from build123d import *

# Parameters (mm, degrees)
CROQUIS1_R              = 10.5
SALIENTE_EXTRUIR1_DEPTH = 10


with BuildPart() as part:
    # Croquis1 → Saliente-Extruir1 (new body)
    with BuildSketch(Plane(origin=(0, 0, 0), x_dir=(0, 0, -1), z_dir=(1, 0, 0))):
        with BuildLine():
            Line((-18.5, 12.5), (18.5, 12.5))
            ThreePointArc((18.5, 12.5), (30.713875068, 2.659183298), (23.696629213, -11.36859907))
            ThreePointArc((23.696629213, -11.36859907), (0, -16.52778731), (-23.696629213, -11.36859907))
            ThreePointArc((-23.696629213, -11.36859907), (-30.713875068, 2.659183298), (-18.5, 12.5))
        make_face()
        with Locations((18.5, 0)):
            Circle(CROQUIS1_R, mode=Mode.SUBTRACT)
        with Locations((-18.5, 0)):
            Circle(CROQUIS1_R, mode=Mode.SUBTRACT)
        with BuildLine():
            Line((-6, -6.020797289), (-6, 6.020797289))
            ThreePointArc((-6, 6.020797289), (0, 8.5), (6, 6.020797289))
            Line((6, 6.020797289), (6, -6.020797289))
            ThreePointArc((6, -6.020797289), (0, -8.5), (-6, -6.020797289))
        make_face(mode=Mode.SUBTRACT)
    extrude(amount=SALIENTE_EXTRUIR1_DEPTH)


solid = part.part
Check sheet for the modelled part. Datum: model origin and axes. Units: mm. A direction names the side the tool comes from. Round coordinates to 2 decimals unless told otherwise and drop trailing zeros. Order: outer loops, then holes, each group sorted by start corner. A loop starts at its lowest first (then second) coordinate and runs counter-clockwise, first axis right, second up.
Q1. Cross-section at B-B, the plane x = 8.75. Enter the section's corners in (y, z).
Filled sheet:
outline: (-11.37, -23.7) arc R12.5 ccw to (12.5, -18.5) - (12.5, 18.5) arc R12.5 ccw to (-11.37, 23.7) arc R57 ccw to start; hole circle Ø21 at (0, -18.5); hole circle Ø21 at (0, 18.5); hole (-6.02, -6) - (6.02, -6) arc R8.5 ccw to (6.02, 6) - (-6.02, 6) arc R8.5 ccw to start
Q2. Draft check along Z on faces 1 (the face through (4.9, 8.5, 0.1)), 2 (the face through (4.93, 2.43, 30.76)), 3 (the face through (10, -2, -7)). Enter one of: pulls with the +Z half, pulls with the -Z half, needs draft (parallel to the pull), parting line crosses it, or undercut.
Filled sheet:
face 1: undercut
face 2: pulls with the +Z half
face 3: needs draft
Q3. Cross-section at A-A, the plane y = 0. Enter the section's corners in (x, z), plus the area to 3 significant figures.
Filled sheet:
outline: (0, -31) - (10, -31) - (10, -29) - (0, -29) - close; (0, -8) - (10, -8) - (10, -6) - (0, -6) - close; (0, 6) - (10, 6) - (10, 8) - (0, 8) - close; (0, 29) - (10, 29) - (10, 31) - (0, 31) - close
area: 80.0 mm2
Q4. Scan lines: L1, parallel to Z at x = 3.5, y = 4.75; L2, parallel to Z at x = 7.5, y = -9.25; L3, parallel to Y at x = 8.75, z = 0. Record each from-to range of solid material in increasing order.
Filled sheet:
L1: z = -30.06 to -27.86, -9.14 to -6, 6 to 9.14, 27.86 to 30.06
L2: z = -26.91 to -23.47, -13.53 to 13.53, 23.47 to 26.91
L3: y = -16.53 to -8.5, 8.5 to 12.5
Q5. Cross-section at C-C, the plane z = -5. Enter the section's corners in (x, y).
Filled sheet:
outline: (0, -16.31) - (10, -16.31) - (10, -6.87) - (0, -6.87) - close; (0, 6.87) - (10, 6.87) - (10, 12.5) - (0, 12.5) - close
Q6. Set-up check for faces 4 (the face through (5, 0, -6)), 5 (the face through (5, 12.5, 0)): record each of +Z, -Z, +X, -X, +Y, -Y from which the full face is reachable in a straight line by a thin tool's end or side.
Filled sheet:
face 4: +X, -X
face 5: +Z, -Z, +X, -X, +Y
Q7. Cross-section at D-D, the plane y = -3.5. Enter the section's corners in (x, z), plus the area to 3 significant figures.
Filled sheet:
outline: (0, -30.5) - (10, -30.5) - (10, -28.4) - (0, -28.4) - close; (0, -8.6) - (10, -8.6) - (10, -6) - (0, -6) - close; (0, 6) - (10, 6) - (10, 8.6) - (0, 8.6) - close; (0, 28.4) - (10, 28.4) - (10, 30.5) - (0, 30.5) - close
area: 94.0 mm2
Q8. Depth check by flat-ended pin: P1, Ø12.5, axis at y = 0, z = 18.5, coming from the +X side; P2, Ø5, axis at x = 1.5, y = 4.5, coming from the +Z side; P3, Ø6, axis at y = -8.5, z = 19.5, coming from the -X side; P4, Ø3, axis at x = 2, y = -7, coming from the +Z side (3 decimals). Enter the tip coordinate at first touch or a pass-through.
Filled sheet:
P1: passes through
P2: stops at z = 30.84
P3: stops at x = 0
P4: stops at z = 29.725
